Check sheet for the modelled part. Datum: model origin and axes. Units: mm. Give positions to 0.01 mm unless a question says otherwise; leave off trailing zeros. Write each loop counter-clockwise with the first axis right and the second up, starting at its lowest first coordinate (ties: lowest second). Pieces come first, ordered by that corner, then holes. Notation, with made-up numbers: (-37, 73) -> (-27, 73) arc R33 cw to (-27, 109) -> close; hole circle Ø9 at (3, 57). An arc over 180 degrees is marked (long way). Return JSON: item names as keys, results as strings.
from build123d import *

# Parameters (mm, degrees)
SKETCH1_R                   = 3.175
SKETCH1_R_2                 = 8
BOSS_EXTRUDE1_DEPTH         = 6.35
FILLET1_R                   = 5
F_1_4_20_TAPPED_HOLE1_D     = 5.1054
F_1_4_20_TAPPED_HOLE1_DEPTH = 19.05
F_1_4_20_TAPPED_HOLE1_TIP   = 1.533816902


with BuildPart() as part:
    # Sketch1 → Boss-Extrude1 (new body)
    with BuildSketch(Plane.XY):
        Polygon((16.184070214, -255.902577388), (-19.05, -235.560177465), (-19.05, -178.2), (19.05, -178.2), (19.05, -255.902577388), align=None)
        with Locations((13.834070214, -246.4)):
            Circle(SKETCH1_R, mode=Mode.SUBTRACT)
        with Locations((0, -203.2)):
            Circle(SKETCH1_R_2, mode=Mode.SUBTRACT)
    extrude(amount=BOSS_EXTRUDE1_DEPTH)

    # Fillet1
    fillet1_edges = [part.edges().sort_by_distance(p)[0] for p in [
        (-19.05, -235.560177465, 3.175),
        (-19.05, -178.2, 3.175),
        (19.05, -178.2, 3.175),
    ]]
    fillet(fillet1_edges, radius=FILLET1_R)

    # 1/4-20 Tapped Hole1
    with Locations(Plane.XY.offset(6.35)):
        with Locations((-11.43, -184.7), (-11.43, -231.16), (11.43, -184.7)):
            Hole(F_1_4_20_TAPPED_HOLE1_D / 2, depth=F_1_4_20_TAPPED_HOLE1_DEPTH)
            with Locations((0, 0, -(F_1_4_20_TAPPED_HOLE1_DEPTH + F_1_4_20_TAPPED_HOLE1_TIP / 2))):  # 118° drill point
                Cone(0, F_1_4_20_TAPPED_HOLE1_D / 2, F_1_4_20_TAPPED_HOLE1_TIP, mode=Mode.SUBTRACT)


solid = part.part
(1) Cross-section at B-B on y = -184.7. Enter the section's corners in (x, z), then the cut area to 3 significant figures.
Reply:
{"outline": "(-19.05, 0) -> (-13.98, 0) -> (-13.98, 6.35) -> (-19.05, 6.35) -> close; (-8.88, 0) -> (8.88, 0) -> (8.88, 6.35) -> (-8.88, 6.35) -> close; (13.98, 0) -> (19.05, 0) -> (19.05, 6.35) -> (13.98, 6.35) -> close", "area": "177 mm^2"}
(2) Cross-section at C-C on x = 0. Enter the section's corners in (y, z).
Reply:
{"outline": "(-246.56, 0) -> (-211.2, 0) -> (-211.2, 6.35) -> (-246.56, 6.35) -> close; (-195.2, 0) -> (-178.2, 0) -> (-178.2, 6.35) -> (-195.2, 6.35) -> close"}
(3) Thickness scan on L1, parallel to X at y = -184.7, z = 4.5; L2, parallel to Y at x = -11, z = 1; L3, parallel to Y at x = -11.43, z = 4.75. Record the ranges inside material, lowest first.
Reply:
{"L1": "-19.05 to -13.98, -8.88 to 8.88, 13.98 to 19.05", "L2": "-240.21 to -233.68, -228.64 to -187.22, -182.18 to -178.2", "L3": "-239.96 to -233.71, -228.61 to -187.25, -182.15 to -178.2"}
(4) Cross-section at A-A on z = 3.5. Enter the section's corners in (x, y) (3 decimals).
Reply:
{"outline": "(-19.05, -232.673) arc R5 ccw to (-16.55, -237.004) -> (16.184, -255.903) -> (19.05, -255.903) -> (19.05, -183.2) arc R5 ccw to (14.05, -178.2) -> (-14.05, -178.2) arc R5 ccw to (-19.05, -183.2) -> close; hole circle Ø5.105 at (-11.43, -231.16); hole circle Ø5.105 at (-11.43, -184.7); hole circle Ø16 at (0, -203.2); hole circle Ø5.105 at (11.43, -184.7); hole circle Ø6.35 at (13.834, -246.4)"}
(5) Cross-section at D-D on y = -231.16. Enter the section's corners in (x, z), then the cut area to 3 significant figures.
Reply:
{"outline": "(-19.05, 0) -> (-13.98, 0) -> (-13.98, 6.35) -> (-19.05, 6.35) -> close; (-8.88, 0) -> (19.05, 0) -> (19.05, 6.35) -> (-8.88, 6.35) -> close", "area": "210 mm^2"}
(6) Release check for a two-part mould opening along X. For faces 1 (the flat face through (0.046, -246.585, 3.131)), 2 (the cylindrical face through (3.69, -210.3, 3.13)), 3 (the flat face through (18, -255.903, 3)), 4 (the flat face through (19.05, -219, 3)) record: pulls with the +X half, pulls with the -X half, needs draft (parallel to the pull), parting line crosses it, or undercut.
Reply:
{"face 1": "pulls with the -X half", "face 2": "undercut", "face 3": "needs draft", "face 4": "pulls with the +X half"}
